```python
from build123d import *

# Parameters (mm, degrees)
F0_R     = 4
F1_DEPTH = 2.5
F2_R     = 4
F3_DEPTH = 15


with BuildPart() as f1:
    # F0 (on Top) → F1 (new body, symmetric)
    with BuildSketch(Plane.XY):
        with BuildLine():
            ThreePointArc((20, -7.5), (27.5, 0), (20, 7.5))
            Line((20, 7.5), (-20, 7.5))
            ThreePointArc((-20, 7.5), (-27.5, 0), (-20, -7.5))
            Line((-20, -7.5), (20, -7.5))
        make_face()
        with Locations((-20, 0)):
            Circle(F0_R, mode=Mode.SUBTRACT)
        with Locations((20, 0)):
            Circle(F0_R, mode=Mode.SUBTRACT)
    extrude(amount=F1_DEPTH, both=True)

    # F2 (on face) → F3 (join)
    with BuildSketch(Plane.XY.offset(2.5)):
        with Locations((-20, 0)):
            Circle(F2_R)
    extrude(amount=-F3_DEPTH)


solid = f1.part
```
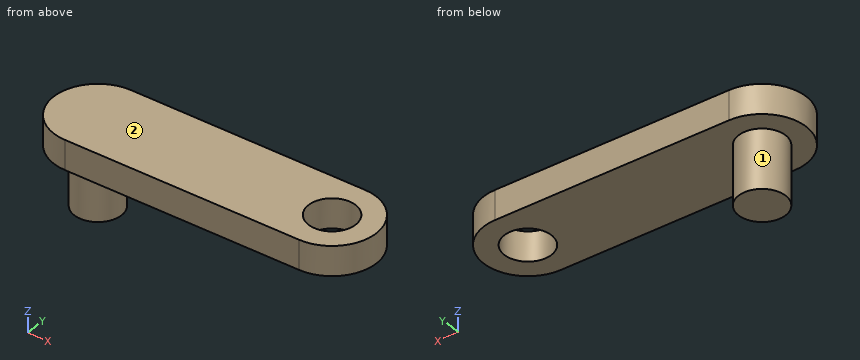
For this review, take the finished solid that the model builds, in its own axes (mm). Face numbers are marked on the shaded views. A direction names the side the tool comes from. Give positions to 0.01 mm unless a question says otherwise; leave off trailing zeros. Loops run counter-clockwise (first coordinate to the right, second up) from the corner with the lowest first, then second, coordinate; pieces in that order, holes last. Notation, with made-up numbers: M 75.5,34 L 120.5,34 A28 cw 120.5,61 Z; hole C 47,89 d6. An arc over 180 degrees is marked long. One line per item, written item: value. Start each with the question number.
Q1. For L1, parallel to Y at x = 20, z = -0.35; L2, parallel to Z at x = 9.5, y = 6; L3, parallel to X at y = -3, z = -4, list the stretches that pass through material, from the lowest coordinate up.
Q2. Machinability: for the marked faces 1 and 2, which of the approach directions +Z, -Z, +X, -X, +Y, -Y give a long, thin tool a straight path to every point of the face, cutting with its end or side? Answer none if there is none.
Q3. Add section D-D (x = 15.5). Give the boundary of the cut face in (y, z), and give its area (3 significant figures).
Q4. Add section B-B (z = -10). Give the boundary of the cut face in (x, y), and give its area (3 significant figures).
Q5. Add section A-A (y = 0). Give the boundary of the cut face in (x, z), and give its area (3 significant figures).
Q6. Add section C-C (y = -3.25). Give the boundary of the cut face in (x, z).
Q7. Clearance check with flat-ended pins moving along their axes: pin 1 Ø5 at (y, z) = (2, -3.5) entering from -X; pin 2 Ø6.5 at (x, y) = (20, 0) entering from -Z; pin 3 Ø1 at (x, y) = (8.5, 1.5) entering from -Z; pin 4 Ø4 at (y, z) = (0, -8.5) entering from +X. State where each tip first meets the part, or that it passes through.
Reply:
1. L1: -7.5 to -4, 4 to 7.5
1. L2: -2.5 to 2.5
1. L3: -22.65 to -17.35
2. face 1: -Z
2. face 2: +Z, +X, -X, +Y, -Y
3. outline: M -7.5,-2.5 L 7.5,-2.5 L 7.5,2.5 L -7.5,2.5 Z
3. area: 75.0 mm²
4. outline: C -20,0 d8
4. area: 50.3 mm²
5. outline: M -27.5,-2.5 L -24,-2.5 L -24,-12.5 L -16,-12.5 L -16,-2.5 L 16,-2.5 L 16,2.5 L -27.5,2.5 Z; M 24,-2.5 L 27.5,-2.5 L 27.5,2.5 L 24,2.5 Z
5. area: 315 mm²
6. outline: M -26.76,-2.5 L -22.33,-2.5 L -22.33,-12.5 L -17.67,-12.5 L -17.67,-2.5 L 17.67,-2.5 L 17.67,2.5 L -26.76,2.5 Z; M 22.33,-2.5 L 26.76,-2.5 L 26.76,2.5 L 22.33,2.5 Z
7. pin 1: x = -27.5
7. pin 2: through
7. pin 3: z = -2.5
7. pin 4: x = -16
